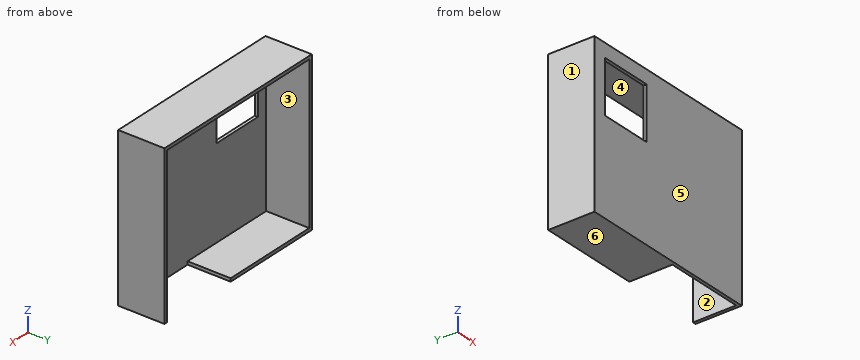
Autodesk Inventor part; units mm, degrees
ref_plane "YZ Plane" through (0, 0, 0) normal (1, 0, 0) x (0, 1, 0)
ref_plane "XZ Plane" through (0, 0, 0) normal (0, 1, 0) x (-1, 0, 0)
ref_plane "XY Plane" through (0, 0, 0) normal (0, 0, 1) x (1, 0, 0)
sketch "Sketch1" plane through (0, 0, 0) normal (0, 1, 0) x (-1, 0, 0)
  line L0 (0, 0) -> (178, 0)
  line L1 (178, 0) -> (178, -152)
  line L2 (178, -152) -> (0, -152)
  line L3 (0, -152) -> (0, 0)
  dimension "d1" = 152
  dimension "d2" = 178
extrude "Extrusion1" add sketch "Sketch1" along normal blind 44
shell "Shell1" thickness 3 removed faces 1 at (-118.6667, 44, -101.3333)
sketch "Sketch3" plane through (0, 0, -152) normal (0, 0, -1) x (-1, 0, 0)
  line L0 (3, 3) -> (3, 44)
  line L1 (0, 44) -> (178, 44)
  line L2 (3, 3) -> (80, 3)
  line L3 (80, 3) -> (80, 44)
  line L4 (80, 44) -> (3, 44)
  line L5 (3, 44) -> (3, 3)
  point P0 (0, 0)
  dimension "d9" = 77
extrude "Extrusion3" cut sketch "Sketch3" against normal blind 4
sketch "Sketch4" plane through (0, 0, 0) normal (0, -1, 0) x (1, 0, 0)
  line L0 (-175, -3) -> (-175, -149)
  line L1 (-175, -3) -> (-165, -3)
  line L2 (-165, -3) -> (-165, -13)
  line L3 (-165, -13) -> (-175, -13)
  line L4 (-175, -13) -> (-175, -3)
  line L5 (-165, -13) -> (-115, -13)
  line L6 (-115, -13) -> (-115, -63)
  line L7 (-115, -63) -> (-165, -63)
  line L8 (-165, -63) -> (-165, -13)
  point P0 (0, 0)
  dimension "d12" = 10
  dimension "d13" = 10
  dimension "d14" = 50
  dimension "d15" = 50
extrude "Extrusion4" cut sketch "Sketch4" against normal blind 4 contours L5 L6 L7 L8
properties part number "back side"
Source: CAD feature listing. Evaluate the final solid. Frame: model axes, mm. Face numbers are marked on the shaded views. A direction names the side the tool comes from. Round coordinates to 2 decimals unless told otherwise and drop trailing zeros. Order: outer loops, then holes, each group sorted by start corner. A loop starts at its lowest first (then second) coordinate and runs counter-clockwise, first axis right, second up. Notation, with made-up numbers: (-19.75, 49) - (35.25, 49) arc R33 ccw to (35.25, 81) - close; hole circle Ø4 at (3, -8.5). An arc over 180 degrees is marked (long way). Use a Markdown table: item, result. Add a question column.
1. Section query A-A (z = -33). Return the cut outline in (x, y), then the cut area to 3 significant figures.
2. Section query D-D (z = -94). Return the cut outline in (x, y).
3. First-contact query: pin 1 (12 mm diameter, centred on x = -105, z = -71, fed in from +Y). Flat tip, straight axial feed; report the tip coordinate or a pass-through.
4. Set-up query: the marked faces 1, 2 and 3. Return all of +Z, -Z, +X, -X, +Y, -Y with unobstructed straight access to the full face (end or side cutting, diameter ignored); none if empty.
5. Line query: probe 1 along X at (y, z) = (41, -120.5); probe 2 along Z at (x, y) = (-123.5, 25); probe 3 along Y at (x, z) = (-8.5, -12). Output: solid intervals per line, ascending.
6. Section query B-B (x = -149.5). Return the cut outline in (y, z), then the cut area to 3 significant figures.
7. Section query C-C (y = 14). Return the cut outline in (x, z), then the cut area to 3 significant figures.
8. Mould query, pull axis Z, two halves, no side actions, for the marked faces 4, 5 and 6. Classes: +Z half, -Z half, draft (parallel to the pull), parting line (faces both ways), or undercut.
Derived:
| question | item | result |
|---|---|---|
| 1 | outline | (-178, 0) - (-165, 0) - (-165, 3) - (-175, 3) - (-175, 44) - (-178, 44) - close; (-115, 0) - (0, 0) - (0, 44) - (-3, 44) - (-3, 3) - (-115, 3) - close |
| 1 | area | 630 mm2 |
| 2 | outline | (-178, 0) - (0, 0) - (0, 44) - (-3, 44) - (-3, 3) - (-175, 3) - (-175, 44) - (-178, 44) - close |
| 3 | pin 1 | y = 3 |
| 4 | face 1 | +Z, -Z, -X, +Y, -Y |
| 4 | face 2 | -Z, +Y |
| 4 | face 3 | +Y |
| 5 | probe 1 | -178 to -175, -3 to 0 |
| 5 | probe 2 | -152 to -149, -3 to 0 |
| 5 | probe 3 | 0 to 3 |
| 6 | outline | (0, -152) - (44, -152) - (44, -149) - (3, -149) - (3, -63) - (0, -63) - close; (0, -13) - (3, -13) - (3, -3) - (44, -3) - (44, 0) - (0, 0) - close |
| 6 | area | 552 mm2 |
| 7 | outline | (-178, -152) - (-80, -152) - (-80, -149) - (-175, -149) - (-175, -3) - (-3, -3) - (-3, -152) - (0, -152) - (0, 0) - (-178, 0) - close |
| 7 | area | 1,710 mm2 |
| 8 | face 4 | undercut |
| 8 | face 5 | draft |
| 8 | face 6 | -Z half |
